CAD build for the part. Positions are in the model's coordinates, mm. Face numbers are marked on the shaded views. A direction names the side the tool comes from. Give positions to 0.01 mm unless a question says otherwise; leave off trailing zeros. Loops run counter-clockwise (first coordinate to the right, second up) from the corner with the lowest first, then second, coordinate; pieces in that order, holes last.
Item 1: Probe probe 1 along Y at (x, z) = (0, 0.85); probe 2 along Y at (x, z) = (17, 1.8); probe 3 along X at (y, z) = (2.25, 1.9). List the from-to ranges inside material, lowest first.
Item 2: Which spindle directions (+Z, -Z, +X, -X, +Y, -Y) get a long thin tool onto all of the face, cutting with end or side? Do the marked faces 1 and 2. Say none if no direction does.
Item 3: Mould opens along Y. For the marked faces 3, 4, 5 and 6 say: released by +Y, released by -Y, zero draft, split by the parting line, or undercut.
Item 4: Saw through at C-C on y = 11.5. Give the cut face in (x, z).
Item 5: Drop flat-ended pins along their axis: P1, Ø2.5, axis at x = -8, y = 0, coming from the +Z side; P2, Ø1, axis at x = 4, z = 2, coming from the -Y side; P3, Ø3.5, axis at x = 0, y = 8, coming from the -Z side. Give the stop position or say it passes through.
Item 6: Saw through at B-B on x = 0. Give the cut face in (y, z), plus the area to 3 significant figures.
Item 7: Saw through at D-D on x = -9. Give the cut face in (y, z).
Item 8: Saw through at A-A on y = 0. Give the cut face in (x, z), plus the area to 3 significant figures.
from build123d import *

# Parameters (mm, degrees)
EXTRUDE_1_DEPTH     = 3
SKETCH_2_R          = 5.15
SKETCH_2_R_2        = 1.5
SKETCH_2_R_3        = 1
CUT_EXTRUDE_1_DEPTH = 3
FILLET_1_R          = 2


with BuildPart() as part:
    # 草图1 → 凸台-拉伸1 (new body)
    with BuildSketch(Plane.XY):
        with BuildLine():
            Line((-17, 8), (-7.549834435, 8))
            ThreePointArc((-7.549834435, 8), (0, -11), (7.549834435, 8))
            Line((7.549834435, 8), (17, 8))
            ThreePointArc((17, 8), (20.5, 11.5), (17, 15))
            Line((17, 15), (-17, 15))
            ThreePointArc((-17, 15), (-20.5, 11.5), (-17, 8))
        make_face()
    extrude(amount=EXTRUDE_1_DEPTH)

    # 草图2 → 切除-拉伸1 (cut)
    with BuildSketch(Plane.XY.offset(3)):
        Circle(SKETCH_2_R)
        with Locations((8, 0)):
            Circle(SKETCH_2_R_2)
        with Locations((0, -8)):
            Circle(SKETCH_2_R_2)
        with Locations((-8, 0)):
            Circle(SKETCH_2_R_2)
        with Locations((0, 8)):
            Circle(SKETCH_2_R_2)
        with Locations((-17, 11.5)):
            Circle(SKETCH_2_R_3)
        with Locations((17, 11.5)):
            Circle(SKETCH_2_R_3)
    extrude(amount=-CUT_EXTRUDE_1_DEPTH, mode=Mode.SUBTRACT)

    # 圆角1
    fillet_1_edges = [part.edges().sort_by_distance(p)[0] for p in [
        (-7.549834435, 8, 1.5),
        (7.549834435, 8, 1.5),
    ]]
    fillet(fillet_1_edges, radius=FILLET_1_R)


solid = part.part
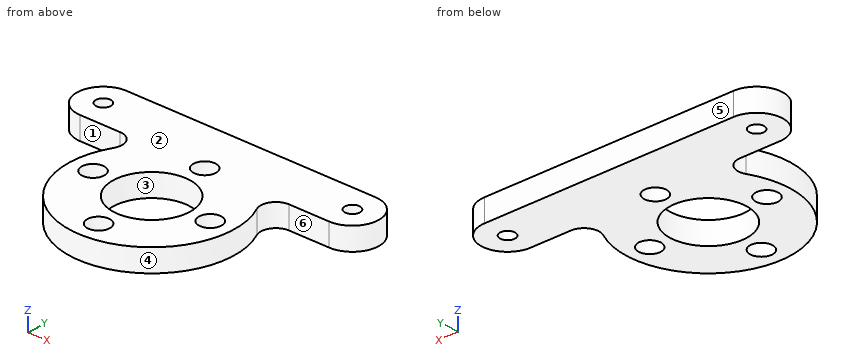
Results below:
1. probe 1: y = -11 to -9.5, -6.5 to -5.15, 5.15 to 6.5, 9.5 to 15
1. probe 2: y = 8 to 10.5, 12.5 to 15
1. probe 3: x = -10.77 to -4.63, 4.63 to 10.77
2. face 1: +Z, -Z, -X, -Y
2. face 2: +Z, +X, -X, +Y, -Y
3. face 3: undercut
3. face 4: undercut
3. face 5: released by +Y
3. face 6: released by -Y
4. outline: (-20.5, 0) - (-18, 0) - (-18, 3) - (-20.5, 3) - close; (-16, 0) - (16, 0) - (16, 3) - (-16, 3) - close; (18, 0) - (20.5, 0) - (20.5, 3) - (18, 3) - close
5. P1: passes through
5. P2: stops at y = -10.43
5. P3: stops at z = 0
6. outline: (-11, 0) - (-9.5, 0) - (-9.5, 3) - (-11, 3) - close; (-6.5, 0) - (-5.15, 0) - (-5.15, 3) - (-6.5, 3) - close; (5.15, 0) - (6.5, 0) - (6.5, 3) - (5.15, 3) - close; (9.5, 0) - (15, 0) - (15, 3) - (9.5, 3) - close
6. area: 29.1 mm2
7. outline: (-6.32, 0) - (-1.12, 0) - (-1.12, 3) - (-6.32, 3) - close; (1.12, 0) - (15, 0) - (15, 3) - (1.12, 3) - close
8. outline: (-11, 0) - (-9.5, 0) - (-9.5, 3) - (-11, 3) - close; (-6.5, 0) - (-5.15, 0) - (-5.15, 3) - (-6.5, 3) - close; (5.15, 0) - (6.5, 0) - (6.5, 3) - (5.15, 3) - close; (9.5, 0) - (11, 0) - (11, 3) - (9.5, 3) - close
8. area: 17.1 mm2
